Answer from the drawing. Dimensions are ordinates in mm from the lowest x, y and z of the part. A direction names the side the tool comes from. Give positions to 0.01 mm unless a question says otherwise; leave off trailing zeros. Order: outer loops, then holes, each group sorted by start corner. A loop starts at its lowest first (then second) coordinate and runs counter-clockwise, first axis right, second up. Notation, with made-up numbers: M 68,55.5 L 116,55.5 A29 ccw 116,83.5 Z; hole C 47,34 d8. An arc over 180 degrees is marked long. One line per item, written item: value.
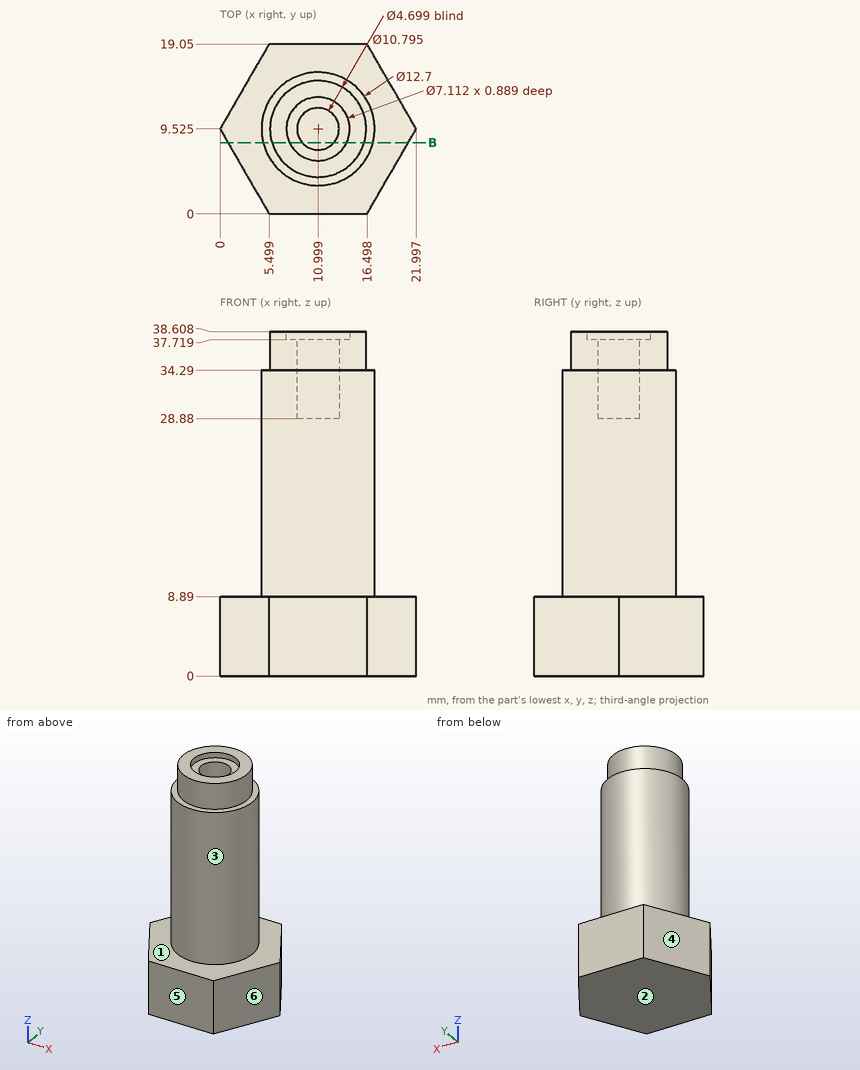
(1) Determine the mould class of the marked faces 3, 4, 5 and 6 for opening direction X: pulls with the +X half, pulls with the -X half, needs draft (parallel to the pull), parting line crosses it, or undercut.
Findings:
face 3: parting line crosses it
face 4: pulls with the -X half
face 5: needs draft
face 6: pulls with the +X half
(2) Section B-B, the plane y = 8 is taken. Give the vertices of the cut face in (x, z) (1 decimal).
Findings:
outline: M 0.9,0 L 21.1,0 L 21.1,8.9 L 17.2,8.9 L 17.2,34.3 L 16.2,34.3 L 16.2,38.6 L 14.2,38.6 L 14.2,37.7 L 12.8,37.7 L 12.8,28.9 L 9.2,28.9 L 9.2,37.7 L 7.8,37.7 L 7.8,38.6 L 5.8,38.6 L 5.8,34.3 L 4.8,34.3 L 4.8,8.9 L 0.9,8.9 Z
(3) Which of the six approach directions +Z, -Z, +X, -X, +Y, -Y give full straight-line access (tool end or side, diameter ignored) to the marked faces 1 and 2?
Findings:
face 1: +Z
face 2: -Z, +X, -X, +Y, -Y
(4) Given P1, Ø2, axis at y = 7, z = 14, coming from the -X side (1 decimal); P2, Ø8, axis at y = 3.5, z = 33, coming from the +X side; P3, Ø10, axis at x = 7.5, z = 23, coming from the +Y side (3 decimals), each flat-ended and moving along its own axis, determine where each tip first touches the part or whether it passes through.
Findings:
P1: stops at x = 4.8
P2: stops at x = 17.02
P3: stops at y = 15.875
(5) Find the intervals of material crossed by probe 1 along Z at (x, y) = (16.25, 1); probe 2 along Z at (x, y) = (11.5, 7); probe 3 along Y at (x, z) = (10.5, 29) (1 decimal), in increasing order. Write a range as from..to.
Findings:
probe 1: z = 0..8.89
probe 2: z = 0..37.72
probe 3: y = 3.2..7.2, 11.8..15.9
